Verification items for the finished model (mm, model axes). A direction names the side the tool comes from. Give positions to 0.01 mm unless a question says otherwise; leave off trailing zeros. Order: outer loops, then holes, each group sorted by start corner. A loop starts at its lowest first (then second) coordinate and runs counter-clockwise, first axis right, second up. Notation, with made-up numbers: (85.25, 13.25) - (128.25, 13.25) arc R34 cw to (128.25, 49.25) - close; hole circle Ø3 at (65.5, 9.25). An arc over 180 degrees is marked (long way). Answer as a JSON object with one key per item and string values.
```python
from build123d import *

# Parameters (mm, degrees)
EXTRUDE_1_DEPTH     = 20
SKETCH_2_R          = 12.5
EXTRUDE_2_DEPTH     = 20
SKETCH_3_R          = 4.5
SKETCH_3_R_2        = 11
CUT_EXTRUDE_1_DEPTH = 105.805216329


with BuildPart() as part:
    # Эскиз1 → Бобышка-Вытянуть1 (new body)
    with BuildSketch(Plane.XY):
        with BuildLine():
            Line((0, 20), (40, 20))
            Line((40, 20), (40, -20))
            Line((40, -20), (0, -20))
            ThreePointArc((0, -20), (-20, 0), (0, 20))
        make_face()
    extrude(amount=EXTRUDE_1_DEPTH)

    # Эскиз2 → Бобышка-Вытянуть2 (add)
    with BuildSketch(Plane.XY):
        with BuildLine():
            ThreePointArc((90.39137509, 14.705321156), (72.358344337, 18.958280561), (78.366684393, 36.484766564))
            Line((78.366684393, 36.484766564), (40, 20))
            Line((40, 20), (40, -20))
            Line((40, -20), (90.39137509, 14.705321156))
        make_face()
        with Locations((83.301270189, 25)):
            Circle(SKETCH_2_R)
    extrude(amount=EXTRUDE_2_DEPTH)

    # Эскиз3 → Вырез-Вытянуть1 (cut, through all)
    with BuildSketch(Plane.XY.offset(20)):
        with BuildLine():
            ThreePointArc((85.551270189, 21.102885683), (79.404155872, 22.75), (81.051270189, 28.897114317))
            Line((81.051270189, 28.897114317), (68.060889132, 21.397114317))
            ThreePointArc((68.060889132, 21.397114317), (72.560889132, 21.397114317), (74.810889132, 17.5))
            ThreePointArc((74.810889132, 17.5), (74.208003449, 15.25), (72.560889132, 13.602885683))
            Line((72.560889132, 13.602885683), (85.551270189, 21.102885683))
        make_face()
        with Locations((83.301270189, 25)):
            Circle(SKETCH_3_R)
        with Locations((20, 0)):
            Circle(SKETCH_3_R_2)
        with Locations((70.310889132, 17.5)):
            Circle(SKETCH_3_R)
    extrude(amount=-CUT_EXTRUDE_1_DEPTH, mode=Mode.SUBTRACT)


solid = part.part
```
(1) Section check D-D (x = 7). Record the cut outline in (y, z).
Computed values:
{"outline": "(-20, 0) - (20, 0) - (20, 20) - (-20, 20) - close"}
(2) Material ranges on line 1 along Y through (x, z) = (20, 4.75); line 2 along Y through (x, z) = (36, 8.25); line 3 along X through (y, z) = (-7, 17.5) (3 decimals), recorded low to high. Write a range as [from, to].
Computed values:
{"line 1": "y = [-20, -11], [11, 20]", "line 2": "y = [-20, 20]", "line 3": "x = [-18.735, 11.515], [28.485, 58.876]"}
(3) Section check C-C (y = 17.5). Record the cut outline in (x, z).
Computed values:
{"outline": "(-9.68, 0) - (65.81, 0) - (65.81, 20) - (-9.68, 20) - close; (79.31, 0) - (93.3, 0) - (93.3, 20) - (79.31, 20) - close"}
(4) Gauge pin test, flat ends, axial feed: pin 1 Ø3 at (y, z) = (9, 6) entering from -X; pin 2 Ø10 at (x, z) = (15.5, 12) entering from +Y; pin 3 Ø6 at (x, z) = (75, 9.5) entering from -Y. Record the tip position at first contact, or that the pin passes through.
Computed values:
{"pin 1": "stops at x = -18.54", "pin 2": "stops at y = 20", "pin 3": "stops at y = 2.04"}
(5) Section check B-B (x = 20). Record the cut outline in (y, z), then the cut area to 3 significant figures.
Computed values:
{"outline": "(-20, 0) - (-11, 0) - (-11, 20) - (-20, 20) - close; (11, 0) - (20, 0) - (20, 20) - (11, 20) - close", "area": "360 mm²"}
(6) Release check for a two-part mould opening along Y. For faces 1 (the cylindrical face through (-20, 0, 10)), 2 (the flat face through (59.452, 28.358, 9.86)), 3 (the cylindrical face through (30.161, -4.213, 10.14)) record: pulls with the +Y half, pulls with the -Y half, needs draft (parallel to the pull), parting line crosses it, or undercut.
Computed values:
{"face 1": "parting line crosses it", "face 2": "pulls with the +Y half", "face 3": "undercut"}
(7) Access from +Z, -Z, +X, -X, +Y, -Y to the whole of each face (thin tool, end or side, straight path). Record for faces 4 (the flat face through (74.65, 25.2, 10.14)), 5 (the flat face through (20, 20, 10)), 6 (the flat face through (64.84, -2.89, 9.86)).
Computed values:
{"face 4": "+Z, -Z", "face 5": "+Z, -Z, -X, +Y", "face 6": "+Z, -Z, +X, -Y"}
(8) Section check A-A (z = 17.5). Record the cut outline in (x, y).
Computed values:
{"outline": "(0, -20) - (40, -20) - (90.39, 14.71) arc R12.5 ccw to (78.37, 36.48) - (40, 20) - (0, 20) arc R20 ccw to start; hole circle Ø22 at (20, 0); hole (68.06, 21.4) arc R4.5 ccw to (72.56, 13.6) - (85.55, 21.1) arc R4.5 ccw to (81.05, 28.9) - close"}
